Build history of the part. All positions in model axes, mm. A direction names the side the tool comes from. Give positions to 0.01 mm unless a question says otherwise; leave off trailing zeros. Order: outer loops, then holes, each group sorted by start corner. A loop starts at its lowest first (then second) coordinate and runs counter-clockwise, first axis right, second up. Notation, with made-up numbers: (-20.75, 33) - (-6.75, 33) arc R16 cw to (-6.75, 39) - close; hole circle Ø3 at (-30.75, 84). An arc over 180 degrees is marked (long way). Write each question's results on one line, items separated by ' | '. Start each with the question number.
from build123d import *

# Parameters (mm, degrees)
BOSS_EXTRUDE5_DEPTH = 10
SKETCH32_W          = 5
SKETCH32_H          = 7
BOSS_EXTRUDE6_DEPTH = 4
SKETCH15_R          = 2
SKETCH15_R_2        = 1.5
CUT_EXTRUDE8_DEPTH  = 51.921508226
CUT_EXTRUDE18_DEPTH = 9
CUT_EXTRUDE19_DEPTH = 51.921508226
SKETCH20_W          = 18.573206134
SKETCH20_H          = 9.890954849
CUT_EXTRUDE12_DEPTH = 51.921508226
SKETCH28_W          = 11
SKETCH28_H          = 1
CUT_EXTRUDE15_DEPTH = 10
SKETCH37_W          = 7
SKETCH37_H          = 5
BOSS_EXTRUDE7_DEPTH = 1
CUT_EXTRUDE11_DEPTH = 9
CUT_EXTRUDE20_DEPTH = 52.749396132
BOSS_EXTRUDE8_START = -1
BOSS_EXTRUDE8_DEPTH = 1
FILLET15_R          = 3
FILLET16_R          = 0.5


with BuildPart() as part:
    # Sketch14 → Boss-Extrude5 (new body)
    with BuildSketch(Plane.XY):
        with BuildLine():
            Line((27, -8.5), (27, 0))
            Line((27, 0), (0, 0))
            Line((0, 0), (0, -14))
            Line((0, -14), (7, -14))
            ThreePointArc((7, -14), (14, -21), (7, -28))
            Line((7, -28), (0, -28))
            Line((0, -28), (0, -42))
            Line((0, -42), (27, -42))
            Line((27, -42), (27, -33.5))
            Line((27, -33.5), (27, -8.5))
        make_face()
    extrude(amount=BOSS_EXTRUDE5_DEPTH)

    # Sketch32 → Boss-Extrude6 (add)
    with BuildSketch(Plane.ZY):
        with Locations((2.5, -10.5)):
            Rectangle(SKETCH32_W, SKETCH32_H)
        with Locations((2.5, -31.5)):
            Rectangle(SKETCH32_W, SKETCH32_H)
    extrude(amount=BOSS_EXTRUDE6_DEPTH)

    # Sketch15 → Cut-Extrude8 (cut, through all)
    with BuildSketch(Plane.XY.offset(10)):
        with Locations((7, -9)):
            Circle(SKETCH15_R)
        with Locations((22.5, -5.5)):
            Circle(SKETCH15_R_2)
        with Locations((22.5, -36.5)):
            Circle(SKETCH15_R_2)
        with Locations((7, -33)):
            Circle(SKETCH15_R)
        with Locations((-8.5, -36.5)):
            Circle(SKETCH15_R_2)
    extrude(amount=-CUT_EXTRUDE8_DEPTH, mode=Mode.SUBTRACT)

    # Sketch33 → Cut-Extrude18 (cut)
    with BuildSketch(Plane.XY.offset(10)):
        with BuildLine():
            Line((-4, -29.85), (3.5, -29.85))
            ThreePointArc((3.5, -29.85), (5.15, -31.5), (3.5, -33.15))
            Line((3.5, -33.15), (-4, -33.15))
            ThreePointArc((-4, -33.15), (-5.65, -31.5), (-4, -29.85))
        make_face()
        with BuildLine():
            Line((-4, -12.15), (3.5, -12.15))
            ThreePointArc((3.5, -12.15), (5.15, -10.5), (3.5, -8.85))
            Line((3.5, -8.85), (-4, -8.85))
            ThreePointArc((-4, -8.85), (-5.65, -10.5), (-4, -12.15))
        make_face()
    extrude(amount=-CUT_EXTRUDE18_DEPTH, mode=Mode.SUBTRACT)

    # Sketch34 → Cut-Extrude19 (cut, through all)
    with BuildSketch(Plane.XY.offset(10)):
        with BuildLine():
            Line((0, -7), (-4.5, -7))
            ThreePointArc((-4.5, -7), (-6, -5.5), (-4.5, -4))
            Line((-4.5, -4), (0, -4))
            ThreePointArc((0, -4), (1.5, -5.5), (0, -7))
        make_face()
        with BuildLine():
            Line((0, -38), (-4, -38))
            ThreePointArc((-4, -38), (-5.5, -36.5), (-4, -35))
            Line((-4, -35), (0, -35))
            ThreePointArc((0, -35), (1.5, -36.5), (0, -38))
        make_face()
    extrude(amount=-CUT_EXTRUDE19_DEPTH, mode=Mode.SUBTRACT)

    # Sketch20 → Cut-Extrude12 (cut, through all)
    with BuildSketch(Plane.XY.offset(10)):
        with Locations((6.713396933, 2.275477425)):
            Rectangle(SKETCH20_W, SKETCH20_H)
    extrude(amount=-CUT_EXTRUDE12_DEPTH, mode=Mode.SUBTRACT)

    # Sketch28 → Cut-Extrude15 (cut)
    with BuildSketch(Plane.XY.offset(10)):
        with Locations((21.5, -0.5)):
            Rectangle(SKETCH28_W, SKETCH28_H)
    extrude(amount=-CUT_EXTRUDE15_DEPTH, mode=Mode.SUBTRACT)

    # Sketch37 → Boss-Extrude7 (add)
    with BuildSketch(Plane.XZ.offset(42)):
        with Locations((14, 2.5)):
            Rectangle(SKETCH37_W, SKETCH37_H)
    extrude(amount=BOSS_EXTRUDE7_DEPTH)

    # Sketch19 → Cut-Extrude11 (cut)
    with BuildSketch(Plane.XY.offset(10)):
        with BuildLine():
            Line((15.65, -33.65), (15.65, -43))
            ThreePointArc((15.65, -43), (14, -44.65), (12.35, -43))
            Line((12.35, -43), (12.35, -33.65))
            ThreePointArc((12.35, -33.65), (14, -32), (15.65, -33.65))
        make_face()
    extrude(amount=-CUT_EXTRUDE11_DEPTH, mode=Mode.SUBTRACT)

    # Sketch35 → Cut-Extrude20 (cut, through all)
    with BuildSketch(Plane.XY.offset(10)):
        with BuildLine():
            Line((11.35, -3), (12.35, -4))
            Line((12.35, -4), (12.35, -14))
            ThreePointArc((12.35, -14), (14, -15.65), (15.65, -14))
            Line((15.65, -14), (15.65, -4))
            Line((15.65, -4), (16.65, -3))
            Line((16.65, -3), (16.828427125, -3))
            ThreePointArc((16.828427125, -3), (18.328427125, -4.5), (19.828427125, -3))
            Line((19.828427125, -3), (19.828427125, -2.5))
            ThreePointArc((19.828427125, -2.5), (20.267766953, -1.439339828), (21.328427125, -1))
            Line((21.328427125, -1), (16, -1))
            Line((16, -1), (16, -2.67))
            Line((16, -2.67), (0, -2.67))
            Line((0, -2.67), (0, -3))
            Line((0, -3), (11.35, -3))
        make_face()
    extrude(amount=-CUT_EXTRUDE20_DEPTH, mode=Mode.SUBTRACT)

    # Sketch39 → Boss-Extrude8 (add)
    with BuildSketch(Plane(origin=(0, 0, 0), x_dir=(-1, 0, 0), z_dir=(0, 0, -1)).offset(BOSS_EXTRUDE8_START)):
        with BuildLine():
            Line((-15.65, -4), (-16.65, -3))
            Line((-16.65, -3), (-11.35, -3))
            Line((-11.35, -3), (-12.35, -4))
            Line((-12.35, -4), (-12.35, -14))
            ThreePointArc((-12.35, -14), (-14, -15.65), (-15.65, -14))
            Line((-15.65, -14), (-15.65, -4))
        make_face()
    extrude(amount=BOSS_EXTRUDE8_DEPTH)

    # Fillet15
    fillet15_edges = [part.edges().sort_by_distance(p)[0] for p in [
        (27, -42, 5),
        (27, -1, 5),
    ]]
    fillet(fillet15_edges, radius=FILLET15_R)

    # Fillet16
    fillet16_edges = [part.edges().sort_by_distance(p)[0] for p in [
        (0, -42, 5),
        (-4, -35, 2.5),
        (-4, -33.15, 3),
        (-4, -29.85, 3),
        (-4, -28, 2.5),
        (-4, -14, 2.5),
        (-4, -7, 2.5),
        (-4, -12.15, 3),
        (-4, -8.85, 3),
        (0, -4, 5),
        (0, -38, 5),
        (10.5, -43, 2.5),
        (17.5, -43, 2.5),
        (15.65, -43, 3),
        (12.35, -43, 3),
        (15.65, -4, 5.5),
        (12.35, -4, 5.5),
        (11.35, -3, 5.5),
    ]]
    fillet(fillet16_edges, radius=FILLET16_R)


solid = part.part
Item 1: Cut at D-D, the plane y = -21. List the corners of the cut face in (x, z), then the cut area to 3 significant figures.
Item 2: Probe line 1 along Y through (x, z) = (22.5, 5.75); line 2 along Y through (x, z) = (7, 3.25); line 3 along Y through (x, z) = (8.5, 1). List the from-to ranges inside material, lowest first. Write a range as from..to.
Item 3: Which spindle directions (+Z, -Z, +X, -X, +Y, -Y) get a long thin tool onto all of the face, cutting with end or side? Do faces 4 (the flat face through (-2, -35, 2)), 5 (the flat face through (1, -33.15, 5)), 6 (the cylindrical face through (14, -32, 6)). Say none if no direction does.
Item 4: Flat gauge pins, fed straight in: pin 1 Ø0.5 at (y, z) = (-3, 6) entering from -X; pin 2 Ø2.5 at (x, y) = (22.5, -5.5) entering from +Z; pin 3 Ø0.8 at (x, y) = (11.5, -42.5) entering from +Z; pin 4 Ø3 at (x, z) = (-1, 1.5) entering from -Y. Where does each tip first touch, or does it go through?
Item 5: Two-plate mould, pull along X, no slides. Class faces 1 (the flat face through (-4, -31.5, 0.8)), 2 (the flat face through (12.35, -9, 6)), 3 (the flat face through (1, -12.15, 5)): +X half, -X half, draft (parallel to the pull), parting line (faces both ways), or undercut.
Item 6: Cut at C-C, the plane z = 7.25. Count the separate pieces of the cut face and the enclosed holes in it, then the cut area to 3 significant figures.
Item 7: Cut at A-A, the plane y = -36.5. List the corners of the cut face in (x, z), then the cut area to 3 significant figures.
Item 8: Cut at B-B, the plane x = 15. List the corners of the cut face in (y, z), then the cut area to 3 significant figures.
Values found:
1) outline: (14, 0) - (27, 0) - (27, 10) - (14, 10) - close | area: 130 mm2
2) line 1: y = -42..-38, -35..-7, -4..-1 | line 2: y = -42..-35, -31..-28, -14..-11, -7..-3 | line 3: y = -42..-34.32, -31.68..-27.84, -14.16..-10.32, -7.68..-3
3) face 4: +Z, -Z, -X, -Y | face 5: +Z, -X | face 6: +Z, -Y
4) pin 1: stops at x = 0 | pin 2: passes through | pin 3: stops at z = 5 | pin 4: stops at y = -42
5) face 1: -X half | face 2: undercut | face 3: draft
6) separate pieces: 1 | enclosed holes: 4 | area: 733 mm2
7) outline: (1.5, 0) - (21, 0) - (21, 10) - (15.65, 10) - (15.65, 1) - (12.35, 1) - (12.35, 10) - (1.5, 10) - close; (24, 0) - (27, 0) - (27, 10) - (24, 10) - close | area: 195 mm2
8) outline: (-43, 0) - (-3, 0) - (-3, 1) - (-15.31, 1) - (-15.31, 10) - (-32.34, 10) - (-32.34, 1) - (-43, 1) - close | area: 193 mm2
